```python
from build123d import *

# Parameters (mm, degrees)
SKETCH1_W           = 40
SKETCH1_H           = 37
BOSS_EXTRUDE1_DEPTH = 19
BOSS_EXTRUDE2_DEPTH = 3
SKETCH3_R           = 6.5
BOSS_EXTRUDE3_DEPTH = 2
SKETCH5_R           = 3
BOSS_EXTRUDE4_DEPTH = 4
SKETCH6_W           = 54
SKETCH6_H           = 19
BOSS_EXTRUDE5_DEPTH = 2
SKETCH7_R           = 2.05
CUT_EXTRUDE1_DEPTH  = 2


with BuildPart() as part:
    # Sketch1 → Boss-Extrude1 (new body)
    with BuildSketch(Plane.XY):
        with Locations((20, 18.5)):
            Rectangle(SKETCH1_W, SKETCH1_H)
    extrude(amount=BOSS_EXTRUDE1_DEPTH)

    # Sketch2 → Boss-Extrude2 (add)
    with BuildSketch(Plane(origin=(0, 37, 0), x_dir=(1, 0, 0), z_dir=(0, 1, 0))):
        with BuildLine():
            Line((7, -0.5), (7, -5))
            ThreePointArc((7, -5), (5, -9.5), (7, -14))
            Line((7, -14), (7, -18.5))
            Line((7, -18.5), (27.458618735, -18.5))
            ThreePointArc((27.458618735, -18.5), (40, -9.5), (27.458618735, -0.5))
            Line((27.458618735, -0.5), (7, -0.5))
        make_face()
    extrude(amount=BOSS_EXTRUDE2_DEPTH)

    # Sketch3 → Boss-Extrude3 (add)
    with BuildSketch(Plane(origin=(0, 40, 0), x_dir=(1, 0, 0), z_dir=(0, 1, 0))):
        with Locations((30.5, -9.5)):
            Circle(SKETCH3_R)
    extrude(amount=BOSS_EXTRUDE3_DEPTH)

    # Sketch5 → Boss-Extrude4 (add)
    with BuildSketch(Plane(origin=(0, 42, 0), x_dir=(1, 0, 0), z_dir=(0, 1, 0))):
        with Locations((30.5, -9.5)):
            Circle(SKETCH5_R)
    extrude(amount=BOSS_EXTRUDE4_DEPTH)

    # Sketch6 → Boss-Extrude5 (add)
    with BuildSketch(Plane(origin=(0, 28.999999912, 0), x_dir=(-1, 0, 0), z_dir=(0, -1, 0))):
        with Locations((-20, -9.5)):
            Rectangle(SKETCH6_W, SKETCH6_H)
    extrude(amount=-BOSS_EXTRUDE5_DEPTH)

    # Sketch7 → Cut-Extrude1 (cut)
    with BuildSketch(Plane(origin=(0, 30.999999912, 0), x_dir=(1, 0, 0), z_dir=(0, 1, 0))):
        with Locations((-4, -4.5)):
            Circle(SKETCH7_R)
        with Locations((-4, -14.5)):
            Circle(SKETCH7_R)
        with Locations((44, -4.5)):
            Circle(SKETCH7_R)
        with Locations((44, -14.5)):
            Circle(SKETCH7_R)
    extrude(amount=-CUT_EXTRUDE1_DEPTH, mode=Mode.SUBTRACT)


solid = part.part
```
Work out the finished part from the listing and answer in its coordinate system (mm). A direction names the side the tool comes from. Round coordinates to 2 decimals unless told otherwise and drop trailing zeros. Write each loop counter-clockwise with the first axis right and the second up, starting at its lowest first coordinate (ties: lowest second). Pieces come first, ordered by that corner, then holes. Notation, with made-up numbers: (24, -38.5) - (40, -38.5) arc R19 cw to (40, -32.5) - close; hole circle Ø8 at (24, -10). An arc over 180 degrees is marked (long way). Return JSON: item names as keys, results as strings. Group by question number.
Q1. Find the intervals of material crossed by L1, parallel to Z at x = 44, y = 30; L2, parallel to X at y = 29.55, z = 4.5; L3, parallel to Y at x = 4, z = 1, in increasing order.
Q2. The part is cut by section D-D on z = 1.5. Write down the section's boundary in (x, y), then the cut area to 3 significant figures.
Q3. For faces 5 (the flat face through (38, 37, 2)), 6 (the cylindrical face through (24.006, 40.986, 9.214)), 7 (the flat face through (17, 38, 18.5)), determine the directions among +Z, -Z, +X, -X, +Y, -Y from which every point of the face is accessible in a straight line to the end or side of a thin tool.
Q4. The part is cut by section A-A on x = 44. Write down the section's boundary in (y, z).
Q5. The mould has two halves that part along X. Classify faces 1 (the flat face through (44, 31, 9)), 2 (the cylindrical face through (39.997, 38.479, 9.752)), 3 (the flat face through (-7, 30, 10)), 4 (the cylindrical face through (-6.05, 30.01, 4.41)): released by +X, released by -X, zero draft, split by the parting line, or undercut.
Q6. The part is cut by section B-B on x = 14. Write down the section's boundary in (y, z), then the cut area to 3 significant figures.
Q7. The part is cut by section C-C on y = 41. Write down the section's boundary in (x, z), then the cut area to 3 significant figures.
Q8. Each of these flat-tipped pins is pushed along its axis until it touches: pin 1 Ø2 at (y, z) = (20.5, 11.5) entering from -X; pin 2 Ø2 at (x, z) = (-3.5, 12.5) entering from +Y; pin 3 Ø1.5 at (y, z) = (39, 16.5) entering from -X; pin 4 Ø3.5 at (x, z) = (-4, 14.5) entering from -Y. Where does it stop, or does it pass through?
Solved:
{
 "1": {"L1": "0 to 2.45, 6.55 to 12.45, 16.55 to 19", "L2": "-7 to -6.05, -1.95 to 41.95, 46.05 to 47", "L3": "0 to 37"},
 "2": {"outline": "(-7, 29) - (0, 29) - (0, 0) - (40, 0) - (40, 29) - (47, 29) - (47, 31) - (40, 31) - (40, 37) - (35.62, 37) - (35.62, 40) - (7, 40) - (7, 37) - (0, 37) - (0, 31) - (-7, 31) - close", "area": "1,590 mm²"},
 "3": {"face 5": "-Z, +X, +Y", "face 6": "+Y", "face 7": "+Z, -X, +Y"},
 "4": {"outline": "(29, 0) - (31, 0) - (31, 2.45) - (29, 2.45) - close; (29, 6.55) - (31, 6.55) - (31, 12.45) - (29, 12.45) - close; (29, 16.55) - (31, 16.55) - (31, 19) - (29, 19) - close"},
 "5": {"face 1": "zero draft", "face 2": "split by the parting line", "face 3": "released by -X", "face 4": "undercut"},
 "6": {"outline": "(0, 0) - (37, 0) - (37, 0.5) - (40, 0.5) - (40, 18.5) - (37, 18.5) - (37, 19) - (0, 19) - close", "area": "757 mm²"},
 "7": {"outline": "circle Ø13 at (30.5, 9.5)", "area": "133 mm²"},
 "8": {"pin 1": "x = 0", "pin 2": "y = 31", "pin 3": "x = 7", "pin 4": "through"}
}
